from build123d import *

# Parameters (mm, degrees)
F0_R     = 2.15265
F0_R_2   = 4
F1_DEPTH = 7.9375
F2_SIZE  = 0.254
F3_R     = 2.15265
F3_R_2   = 4
F3_R_3   = 2.4125
F4_DEPTH = 1.5875


with BuildPart() as f1:
    # F0 (on Top) → F1 (new body)
    with BuildSketch(Plane.XY):
        with BuildLine():
            Line((10.0737161198, 4.5784406229), (1.9754279601, 6.8977031956))
            ThreePointArc((1.9754279601, 6.8977031956), (0, 7.175), (-1.9754279601, 6.8977031956))
            Line((-1.9754279601, 6.8977031956), (-10.0737161198, 4.5784406229))
            ThreePointArc((-10.0737161198, 4.5784406229), (-13.525, 0), (-10.0737161198, -4.5784406229))
            Line((-10.0737161198, -4.5784406229), (-1.9754279601, -6.8977031956))
            ThreePointArc((-1.9754279601, -6.8977031956), (0, -7.175), (1.9754279601, -6.8977031956))
            Line((1.9754279601, -6.8977031956), (10.0737161198, -4.5784406229))
            ThreePointArc((10.0737161198, -4.5784406229), (13.525, 0), (10.0737161198, 4.5784406229))
        make_face()
        with Locations((-8.7625, 0)):
            Circle(F0_R, mode=Mode.SUBTRACT)
        Circle(F0_R_2, mode=Mode.SUBTRACT)
        with Locations((8.7625, 0)):
            Circle(F0_R, mode=Mode.SUBTRACT)
    extrude(amount=F1_DEPTH)

    # F2
    f2_edges = [f1.edges().sort_by_distance(p)[0] for p in [
        (-4, 0, 7.9375),
    ]]
    chamfer(f2_edges, length=F2_SIZE)

    # F3 (on face) → F4 (join)
    with BuildSketch(Plane(origin=(0, 0, 0), x_dir=(1, 0, 0), z_dir=(0, 0, -1))):
        with BuildLine():
            ThreePointArc((10.0737161198, -4.5784406229), (13.525, 0), (10.0737161198, 4.5784406229))
            Line((10.0737161198, 4.5784406229), (1.9754279601, 6.8977031956))
            ThreePointArc((1.9754279601, 6.8977031956), (0, 7.175), (-1.9754279601, 6.8977031956))
            Line((-1.9754279601, 6.8977031956), (-10.0737161198, 4.5784406229))
            ThreePointArc((-10.0737161198, 4.5784406229), (-13.525, 0), (-10.0737161198, -4.5784406229))
            Line((-10.0737161198, -4.5784406229), (-1.9754279601, -6.8977031956))
            ThreePointArc((-1.9754279601, -6.8977031956), (0, -7.175), (1.9754279601, -6.8977031956))
            Line((1.9754279601, -6.8977031956), (10.0737161198, -4.5784406229))
        make_face()
        with Locations((-8.7625, 0)):
            Circle(F3_R, mode=Mode.SUBTRACT)
        Circle(F3_R_2, mode=Mode.SUBTRACT)
        with Locations((8.7625, 0)):
            Circle(F3_R, mode=Mode.SUBTRACT)
        Circle(F3_R_2)
        Circle(F3_R_3, mode=Mode.SUBTRACT)
    extrude(amount=F4_DEPTH)


solid = f1.part
Geometry check sheet. Reference: the model listing, model coordinates, mm. A direction names the side the tool comes from. Give positions to 0.01 mm unless a question says otherwise; leave off trailing zeros.
1) Gauge pin test, flat ends, axial feed: pin 1 (2 mm diameter, centred on y = 2, z = 1.5, fed in from +X); pin 2 (3 mm diameter, centred on x = -9.5, z = 0.5, fed in from -Y); pin 3 (5 mm diameter, centred on y = -4.5, z = -0.5, fed in from -X). Record the tip position at first contact, or that the pin passes through.
Results are:
pin 1: stops at x = 13.42
pin 2: stops at y = -5.17
pin 3: stops at x = -13.08
2) Draft check along X on faces 1 (the cylindrical face through (-0.028, 7.175, 3.242)), 2 (the cylindrical face through (-13.524, -0.086, 3.242)), 3 (the cylindrical face through (-9.043, -2.134, 3.242)), 4 (the cylindrical face through (6.61, -0.09, 3.24)). Enter one of: released by +X, released by -X, zero draft, split by the parting line, or undercut.
Results are:
face 1: split by the parting line
face 2: released by -X
face 3: undercut
face 4: undercut
3) Material ranges on probe 1 along Y at (x, z) = (0, -0.5) (1 decimal); probe 2 along Y at (x, z) = (0, 6) (3 decimals); probe 3 along X at (y, z) = (3, 0.25), recorded low to high.
Results are:
probe 1: y = -7.2 to -2.4, 2.4 to 7.2
probe 2: y = -7.175 to -4, 4 to 7.175
probe 3: x = -12.46 to -2.65, 2.65 to 12.46
4) Cross-section at A-A (y = 0). Give the number of separate pieces and of enclosed holes in the cut face, then the cut area to 3 significant figures.
Results are:
separate pieces: 4
enclosed holes: 0
area: 104 mm2
5) Tool access check on faces 5 (the cylindrical face through (-0.867, -3.905, 3.788)), 6 (the cylindrical face through (13.524, 0.086, 3.242)). Record the directions out of +Z, -Z, +X, -X, +Y, -Y that give a thin tool (end or side, any length) a straight path to the whole face; none if there is none.
Results are:
face 5: +Z
face 6: +Z, -Z, +X
